Input: part model. Units: mm. Frame: model coordinates. Round coordinates to 2 decimals unless told otherwise and drop trailing zeros. Write item = value, one per line.
```python
from build123d import *

# Parameters (mm, degrees)
SKETCH3_W         = 0.762
SKETCH3_H         = 0.254
SKETCH4_R         = 0.44831
SKETCH8_R         = 0.44831
SKETCH9_R         = 0.44831
SKETCH10_R        = 0.44831
SKETCH5_R         = 0.1016
PIN_LNA_END_DEPTH = 2.54
SKETCH15_R        = 0.3429
EXTRUDE1_DEPTH    = 0.0508
CIRPATTERN3_COUNT = 4
SKETCH12_R        = 0.03556
CIRPATTERN1_COUNT = 4


with BuildPart() as part:
    # Sketch3 → Revolve1 (revolve)
    with BuildSketch(Plane(origin=(0, 0, 0), x_dir=(0, 0, -1), z_dir=(1, 0, 0)), mode=Mode.PRIVATE) as revolve1_sk:
        with Locations((22.0726, 0.8128)):
            Rectangle(SKETCH3_W, SKETCH3_H)
    revolve(revolve1_sk.sketch.rotate(Axis((0, 0, -48.3616), (0, 0, 1)), 90), axis=Axis((0, 0, -48.3616), (0, 0, 1)))



with BuildPart() as body_2:
    # SW-00 Coax Jacket X Upper: sweep along a curve in space
    with BuildLine() as sw_00_coax_jacket_x_upper_path:
        Line((4.953, 7.3406, -186.055), (4.953, 7.3406, -178.435))
        Line((4.953, 7.3406, -178.435), (2.872478847, 7.3406, -161.301296391))
        ThreePointArc((2.763684005, 7.294574808, -160.006293151), (2.806048613, 7.329086153, -160.65439699), (2.872478847, 7.3406, -161.301296391))
        Line((2.763684005, 7.294574808, -160.006293151), (0.025075798, 3.13686962, -101.405085392))
        ThreePointArc((0.025075798, 3.13686962, -101.405085392), (0.006271765, 3.108321679, -100.868025718), (0, 3.0988, -100.33))
        Line((0, 3.0988, -100.33), (0, 3.0988, -84.455))
        Line((0, 3.0988, -84.455), (-0.5842, 0.5842, -48.3616))
        Line((-0.5842, 0.5842, -48.3616), (-0.5842, 0.5842, -16.6116))
    # Sketch4 → SW-00 Coax Jacket X Upper (sweep)
    with BuildSketch(Plane.XY.offset(-186.055)):
        with Locations((4.953, 7.3406)):
            Circle(SKETCH4_R)
    sweep(path=sw_00_coax_jacket_x_upper_path.line, transition=Transition.RIGHT)


with BuildPart() as part_1:
    add(part.part)

    add(body_2.part)  # SW-00 Coax Jacket X Lower merges body 2
    # SW-00 Coax Jacket X Lower: sweep along a curve in space
    with BuildLine() as sw_00_coax_jacket_x_lower_path:
        Line((6.223, 7.3406, -186.055), (6.223, 7.3406, -178.435))
        Line((6.223, 7.3406, -178.435), (4.064, 7.3406, -160.655))
        ThreePointArc((4.064, 7.3406, -160.655), (3.988053628, 7.232475572, -159.545590881), (4.031608054, 6.913332282, -158.475778791))
        Line((4.031608054, 6.913332282, -158.475778791), (6.240542312, -2.093682069, -136.351317112))
        ThreePointArc((6.240542312, -2.093682069, -136.351317112), (6.267702876, -2.431735493, -135.236611628), (6.134598563, -2.558955326, -134.08609675))
        Line((6.134598563, -2.558955326, -134.08609675), (0.084425486, -3.091370557, -101.254064355))
        ThreePointArc((0, -3.0988, -100.33), (0.021150572, -3.09693875, -100.793971387), (0.084425486, -3.091370557, -101.254064355))
        Line((0, -3.0988, -100.33), (0, -3.0988, -84.455))
        Line((0, -3.0988, -84.455), (0.5842, -0.5842, -48.3616))
        Line((0.5842, -0.5842, -48.3616), (0.5842, -0.5842, -16.6116))
    # Sketch8 → SW-00 Coax Jacket X Lower (sweep)
    with BuildSketch(Plane.XY.offset(-186.055)):
        with Locations((6.223, 7.3406)):
            Circle(SKETCH8_R)
    sweep(path=sw_00_coax_jacket_x_lower_path.line, transition=Transition.RIGHT)

    # Sweep3: sweep along a curve in space
    with BuildLine() as sweep3_path:
        Line((-6.223, -7.3406, -186.055), (-6.223, -7.3406, -178.435))
        Line((-6.223, -7.3406, -178.435), (-4.064, -7.3406, -160.655))
        ThreePointArc((-4.064, -7.3406, -160.655), (-4.044744837, -7.334400574, -160.452194223), (-4.036200061, -7.315842211, -160.249408743))
        Line((-4.036200061, -7.315842211, -160.249408743), (-3.0988, 0, -100.33))
        Line((-3.0988, 0, -100.33), (-3.0988, 0, -84.455))
        Line((-3.0988, 0, -84.455), (-0.5842, -0.5842, -48.3616))
        Line((-0.5842, -0.5842, -48.3616), (-0.5842, -0.5842, -16.6116))
    # Sketch9 → Sweep3 (sweep)
    with BuildSketch(Plane.XY.offset(-186.055)):
        with Locations((-6.223, -7.3406)):
            Circle(SKETCH9_R)
    sweep(path=sweep3_path.line, transition=Transition.RIGHT)

    # Sweep4: sweep along a curve in space
    with BuildLine() as sweep4_path:
        Line((-4.953, -7.3406, -186.055), (-4.953, -7.3406, -178.435))
        Line((-4.953, -7.3406, -178.435), (-2.794, -7.3406, -160.655))
        ThreePointArc((-2.794, -7.3406, -160.655), (-2.634137004, -7.277961709, -159.764314499), (-2.377457069, -7.092043967, -158.914402504))
        Line((-2.377457069, -7.092043967, -158.914402504), (5.900349004, -0.365392188, -136.473966054))
        ThreePointArc((5.900349004, -0.365392188, -136.473966054), (6.20364645, -0.092905525, -135.223267542), (6.224050743, 0, -133.911231978))
        Line((6.224050743, 0, -133.911231978), (3.12096799, 0, -100.804062615))
        ThreePointArc((3.12096799, 0, -100.804062615), (3.104345024, 0, -100.567290319), (3.0988, 0, -100.33))
        Line((3.0988, 0, -100.33), (3.0988, 0, -84.455))
        Line((3.0988, 0, -84.455), (0.5842, 0.5842, -48.3616))
        Line((0.5842, 0.5842, -48.3616), (0.5842, 0.5842, -16.6116))
    # Sketch10 → Sweep4 (sweep)
    with BuildSketch(Plane.XY.offset(-186.055)):
        with Locations((-4.953, -7.3406)):
            Circle(SKETCH10_R)
    sweep(path=sweep4_path.line, transition=Transition.RIGHT)

    # Sketch5 → Pin LNA End (add)
    with BuildSketch(Plane.XY.offset(-186.055)):
        with Locations((4.953, 7.3406)):
            Circle(SKETCH5_R)
        with Locations((6.223, 7.3406)):
            Circle(SKETCH5_R)
        with Locations((-4.953, -7.3406)):
            Circle(SKETCH5_R)
        with Locations((-6.223, -7.3406)):
            Circle(SKETCH5_R)
    extrude(amount=-PIN_LNA_END_DEPTH)

    # Sketch15 → Extrude1 (cut)
    with BuildSketch(Plane.XY.offset(-16.6116)):
        with Locations((-0.5842, 0.5842)):
            Circle(SKETCH15_R)
    extrude1 = extrude(amount=-EXTRUDE1_DEPTH, mode=Mode.SUBTRACT)

    # CirPattern3: Extrude1 ×4 about axis
    cirpattern3_axis = Axis((0, 0, 0), (0, 0, 1))
    for i in range(1, CIRPATTERN3_COUNT):
        add(extrude1.rotate(cirpattern3_axis, i * 360 / CIRPATTERN3_COUNT), mode=Mode.SUBTRACT)

    # Sweep5: sweep along a path in Sketch11
    with BuildLine(Plane(origin=(0, 0, 0), x_dir=(0, 0, -1), z_dir=(0.7071067811865459, 0.7071067811865491, 0))) as sweep5_path:
        Line((15.7988, 0.826183563), (16.6116, 0.826183563))
        Line((16.6116, 0.826183563), (17.229183431, 0.826183563))
    # Sketch12 → Sweep5 (sweep)
    with BuildSketch(Plane.XY.offset(-16.6624)):
        with Locations((-0.5842, 0.5842)):
            Circle(SKETCH12_R)
    sweep5 = sweep(path=sweep5_path.line)

    # CirPattern1: Sweep5 ×4 about axis
    cirpattern1_axis = Axis((0, 0, 4.39213043), (0, 0, -1))
    for i in range(1, CIRPATTERN1_COUNT):
        add(sweep5.rotate(cirpattern1_axis, i * 360 / CIRPATTERN1_COUNT))


solid = part_1.part
```
1) First-contact query: P1, Ø1, axis at y = -4.5, z = -103.5, coming from the +X side; P2, Ø2, axis at x = -2, y = 0.5, coming from the +Z side; P3, Ø1.5, axis at x = 0.5, z = -149, coming from the -Y side. Flat tips, straight axial feed; report the tip coordinate or a pass-through.
Solutions:
P1 = through
P2 = -16.61
P3 = -4.77
2) Cut plane A-A (z = -66). Count the separate pieces of the cut face and the enclosed holes in it, and give its area (3 significant figures).
Solutions:
separate_pieces = 4
enclosed_holes = 0
area = 2.53 mm^2
3) Draft query along Z for faces 1 (the face through (-3.436, -7.206, -169.485)), 2 (the face through (1.802, 5.322, -130.266)). Return one class per face: +Z half, -Z half, draft (parallel to the pull), parting line (faces both ways), or undercut.
Solutions:
face_1 = undercut
face_2 = parting line
4) Line query: L1, parallel to Y at x = 0.5, z = -48.5; L2, parallel to Y at x = -1, z = -58; L3, parallel to X at y = -4.5, z = -151. Output: solid intervals per line, ascending. Write a range as from..to.
Solutions:
L1 = -1.04..-0.15, 0.14..1.02
L2 = -0.8..-0.06
L3 = 0.14..0.98
